Model file for the job. Use its own axes, mm. A direction names the side the tool comes from. Round coordinates to 2 decimals unless told otherwise and drop trailing zeros. Order: outer loops, then holes, each group sorted by start corner. A loop starts at its lowest first (then second) coordinate and runs counter-clockwise, first axis right, second up. Notation, with made-up numbers: M 54.5,-37 L 110.5,-37 A23 cw 110.5,-3 Z; hole C 77,58 d5. An arc over 180 degrees is marked long. Return JSON: item names as keys, results as strings. Group by question number.
Item 1: Slice it at A-A on y = 0. Write the cut outline in (x, z).
Item 2: Slice it at C-C on z = -70.5. Give the number of separate pieces and of enclosed holes in the cut face, then the cut area to 3 significant figures.
Item 3: Pin check, flat tips, straight feed: pin 1 Ø4 at (x, y) = (15, -15) entering from -Z; pin 2 Ø8.5 at (y, z) = (2, -65.5) entering from -X; pin 3 Ø0.9 at (x, z) = (18, -137.5) entering from -Y; pin 4 Ø0.9 at (y, z) = (-18, -84.5) entering from +X. Stop position of each tip, or through.
Item 4: Pull direction Y, two halves, no side cores. Call faces 1 (the face through (-11, -20, -99)), 2 (the face through (20, -11, -99)), 3 (the face through (8.5, 0, -99)): pulls with the +Y half, pulls with the -Y half, needs draft (parallel to the pull), parting line crosses it, or undercut.
Item 5: Which spindle directions (+Z, -Z, +X, -X, +Y, -Y) get a long thin tool onto all of the face, cutting with end or side? Do faces 4 (the face through (-20, -10, -99)), 5 (the face through (0, -8.5, -99)), 6 (the face through (5.82, 8.87, -98.6)). Say none if no direction does.
Item 6: Probe line 1 along Y through (x, z) = (15, -152); line 2 along Y through (x, z) = (-10, -152). List the from-to ranges inside material, lowest first.
Autodesk Inventor part; units mm, degrees
ref_plane "side_4d_XY" through (-20, 0, -330) normal (-1, 0, 0) x (0, 1, 0)
ref_plane "side_4d_YZ" through (-20, 0, -330) normal (0, 1, 0) x (0, 0, -1)
ref_plane "side_4d_ZX" through (-20, 0, -330) normal (0, 0, -1) x (-1, 0, 0)
sketch "Skizze_1" plane through (0, 0, 0) normal (0, 0, 1) x (1, 0, 0)
  arc A0 (-20, -17) -> (-17, -20) centre (-17, -17) ccw
  line L0 (-17, -20) -> (-4.1, -20)
  line L1 (-4.1, -20) -> (-4.1, -17)
  line L2 (-4.1, -17) -> (-10.5, -17)
  line L3 (-10.5, -17) -> (-10.5, -13.6627)
  arc A1 (-10.0314, -12.5314) -> (-10.5, -13.6627) centre (-8.9002, -13.6627) ccw
  line L4 (-10.0314, -12.5314) -> (-7.4645, -9.9645)
  arc A2 (-3.9289, -8.5) -> (-7.4645, -9.9645) centre (-3.9289, -13.5) ccw
  line L5 (-3.9289, -8.5) -> (3.9289, -8.5)
  arc A3 (7.4645, -9.9645) -> (3.9289, -8.5) centre (3.9289, -13.5) ccw
  line L6 (7.4645, -9.9645) -> (10.0314, -12.5314)
  arc A4 (10.5, -13.6627) -> (10.0314, -12.5314) centre (8.9002, -13.6627) ccw
  line L7 (10.5, -13.6627) -> (10.5, -17)
  line L8 (10.5, -17) -> (4.1, -17)
  line L9 (4.1, -17) -> (4.1, -20)
  line L10 (4.1, -20) -> (17, -20)
  arc A5 (17, -20) -> (20, -17) centre (17, -17) ccw
  line L11 (20, -17) -> (20, -4.1)
  line L12 (20, -4.1) -> (17, -4.1)
  line L13 (17, -4.1) -> (17, -10.5)
  line L14 (17, -10.5) -> (13.6627, -10.5)
  arc A6 (12.5314, -10.0314) -> (13.6627, -10.5) centre (13.6627, -8.9002) ccw
  line L15 (12.5314, -10.0314) -> (9.9645, -7.4645)
  arc A7 (8.5, -3.9289) -> (9.9645, -7.4645) centre (13.5, -3.9289) ccw
  line L16 (8.5, -3.9289) -> (8.5, 3.9289)
  arc A8 (9.9645, 7.4645) -> (8.5, 3.9289) centre (13.5, 3.9289) ccw
  line L17 (9.9645, 7.4645) -> (12.5314, 10.0314)
  arc A9 (13.6627, 10.5) -> (12.5314, 10.0314) centre (13.6627, 8.9002) ccw
  line L18 (13.6627, 10.5) -> (17, 10.5)
  line L19 (17, 10.5) -> (17, 4.1)
  line L20 (17, 4.1) -> (20, 4.1)
  line L21 (20, 4.1) -> (20, 17)
  arc A10 (20, 17) -> (17, 20) centre (17, 17) ccw
  line L22 (17, 20) -> (4.1, 20)
  line L23 (4.1, 20) -> (4.1, 17)
  line L24 (4.1, 17) -> (10.5, 17)
  line L25 (10.5, 17) -> (10.5, 13.6627)
  arc A11 (10.0314, 12.5314) -> (10.5, 13.6627) centre (8.9002, 13.6627) ccw
  line L26 (10.0314, 12.5314) -> (7.4645, 9.9645)
  arc A12 (3.9289, 8.5) -> (7.4645, 9.9645) centre (3.9289, 13.5) ccw
  line L27 (3.9289, 8.5) -> (-3.9289, 8.5)
  arc A13 (-7.4645, 9.9645) -> (-3.9289, 8.5) centre (-3.9289, 13.5) ccw
  line L28 (-7.4645, 9.9645) -> (-10.0314, 12.5314)
  arc A14 (-10.5, 13.6627) -> (-10.0314, 12.5314) centre (-8.9002, 13.6627) ccw
  line L29 (-10.5, 13.6627) -> (-10.5, 17)
  line L30 (-10.5, 17) -> (-4.1, 17)
  line L31 (-4.1, 17) -> (-4.1, 20)
  line L32 (-4.1, 20) -> (-17, 20)
  arc A15 (-17, 20) -> (-20, 17) centre (-17, 17) ccw
  line L33 (-20, 17) -> (-20, 4.1)
  line L34 (-20, 4.1) -> (-17, 4.1)
  line L35 (-17, 4.1) -> (-17, 10.5)
  line L36 (-17, 10.5) -> (-13.6627, 10.5)
  arc A16 (-12.5314, 10.0314) -> (-13.6627, 10.5) centre (-13.6627, 8.9002) ccw
  line L37 (-12.5314, 10.0314) -> (-9.9645, 7.4645)
  arc A17 (-8.5, 3.9289) -> (-9.9645, 7.4645) centre (-13.5, 3.9289) ccw
  line L38 (-8.5, 3.9289) -> (-8.5, -3.9289)
  arc A18 (-9.9645, -7.4645) -> (-8.5, -3.9289) centre (-13.5, -3.9289) ccw
  line L39 (-9.9645, -7.4645) -> (-12.5314, -10.0314)
  arc A19 (-13.6627, -10.5) -> (-12.5314, -10.0314) centre (-13.6627, -8.9002) ccw
  line L40 (-13.6627, -10.5) -> (-17, -10.5)
  line L41 (-17, -10.5) -> (-17, -4.1)
  line L42 (-17, -4.1) -> (-20, -4.1)
  line L43 (-20, -4.1) -> (-20, -17)
  circle A20 centre (0, 0) radius 6
extrude "Extrusion1" add sketch "Skizze_1" against normal blind 200
sketch "Sketch2" plane through (0, 0, 0) normal (0, 0, 1) x (1, 0, 0)
  point P0 (-15, -15)
hole "Drilling 1" at (-15, -15, 0) direction (0, 0, -1) diameter 5 depth 6000
sketch "Sketch3" plane through (0, 0, 0) normal (0, 0, 1) x (1, 0, 0)
  point P0 (15, -15)
hole "Drilling 2" at (15, -15, 0) direction (0, 0, -1) diameter 5 depth 6000
sketch "Sketch4" plane through (0, 0, 0) normal (0, 0, 1) x (1, 0, 0)
  point P0 (15, 15)
hole "Drilling 3" at (15, 15, 0) direction (0, 0, -1) diameter 5 depth 6000
sketch "Sketch5" plane through (0, 0, 0) normal (0, 0, 1) x (1, 0, 0)
  point P0 (-15, 15)
hole "Drilling 4" at (-15, 15, 0) direction (0, 0, -1) diameter 5 depth 6000
ref_plane "side_4d_XY" through (-20, 0, -330) normal (-1, 0, 0) x (0, 1, 0)
ref_plane "side_4d_YZ" through (-20, 0, -330) normal (0, 1, 0) x (0, 0, -1)
ref_plane "side_4d_ZX" through (-20, 0, -330) normal (0, 0, -1) x (-1, 0, 0)
ref_plane "side_1a_XY" through (0, 20, -330) normal (0, 1, 0) x (1, 0, 0)
ref_plane "side_1a_YZ" through (0, 20, -330) normal (1, 0, 0) x (0, 0, -1)
ref_plane "side_1a_ZX" through (0, 20, -330) normal (0, 0, -1) x (0, 1, 0)
ref_plane "side_2b_XY" through (20, 0, -330) normal (1, 0, 0) x (0, -1, 0)
ref_plane "side_2b_YZ" through (20, 0, -330) normal (0, -1, 0) x (0, 0, -1)
ref_plane "side_2b_ZX" through (20, 0, -330) normal (0, 0, -1) x (1, 0, 0)
ref_plane "side_3c_XY" through (0, -20, -330) normal (0, -1, 0) x (-1, 0, 0)
ref_plane "side_3c_YZ" through (0, -20, -330) normal (-1, 0, 0) x (0, 0, -1)
ref_plane "side_3c_ZX" through (0, -20, -330) normal (0, 0, -1) x (0, -1, 0)
ref_plane "end_XY" through (0, 0, -660) normal (0, 0, -1) x (1, 0, 0)
ref_plane "end_YZ" through (0, 0, -660) normal (1, 0, 0) x (0, -1, 0)
ref_plane "end_ZX" through (0, 0, -660) normal (0, -1, 0) x (0, 0, -1)
ref_plane "start_XY" through (0, 0, 0) normal (0, 0, 1) x (1, 0, 0)
ref_plane "start_YZ" through (0, 0, 0) normal (1, 0, 0) x (0, 1, 0)
ref_plane "start_ZX" through (0, 0, 0) normal (0, 1, 0) x (0, 0, 1)
properties part number "MayTec 1.11.040040.43S_Profile 40x40, 4E, S_660_Detail_(0;0,0,0)"
Output values:
{
 "1": {"outline": "M -8.5,-200 L -6,-200 L -6,0 L -8.5,0 Z; M 6,-200 L 8.5,-200 L 8.5,0 L 6,0 Z"},
 "2": {"separate pieces": "1", "enclosed holes": "5", "area": "674 mm²"},
 "3": {"pin 1": "through", "pin 2": "x = -20", "pin 3": "y = -19.95", "pin 4": "x = 19.95"},
 "4": {"face 1": "pulls with the -Y half", "face 2": "needs draft", "face 3": "undercut"},
 "5": {"face 4": "+Z, -Z, -X, +Y, -Y", "face 5": "+Z, -Z, -Y", "face 6": "+Z, -Z"},
 "6": {"line 1": "-20 to -17.5, -12.5 to -10.5, 10.5 to 12.5, 17.5 to 20", "line 2": "-20 to -17, -12.5 to -7.5, 7.5 to 12.5, 17 to 20"}
}
